Verification items for the finished model (mm, model axes). A direction names the side the tool comes from. Give positions to 0.01 mm unless a question says otherwise; leave off trailing zeros. Loops run counter-clockwise (first coordinate to the right, second up) from the corner with the lowest first, then second, coordinate; pieces in that order, holes last. Notation, with made-up numbers: (-26, -8.5) - (-8, -8.5) arc R14 cw to (-8, 4.5) - close; hole circle Ø4 at (58.25, 78.5). An arc over 180 degrees is marked (long way). Answer in a Markdown table with one row per item.
```python
from build123d import *

# Parameters (mm, degrees)
SKETCH1_W                          = 38.1
SKETCH1_H                          = 63.5
MAIN_BODY_DEPTH                    = 3.175
SKETCH2_W                          = 3.2258
SKETCH2_H                          = 6.35
TABS_DEPTH                         = 3.175
SKETCH5_R                          = 0.508
MOTOR_CUT_DEPTH                    = 4.175
SKETCH6_R                          = 3.2385
CUT_FOR_AXLE_DEPTH                 = 4.175
ROUND_OFF_BACK_CORNER_DEPTH        = 4.175
SKETCH8_W                          = 3.2258
SKETCH8_H                          = 6.35
CUT_FOR_TABS_DEPTH                 = 4.175
SKETCH9_R                          = 1.5875
CUT_FOR_BRACKET_SCREW_DEPTH        = 4.175
SKETCH10_R                         = 3.048
CUT_FOR_BASIC_2ND_MOUNT_AXLE_DEPTH = 4.175
SKETCH11_W                         = 9.398
SKETCH11_H                         = 5.08
CUT_EXTRUDE1_DEPTH                 = 4.175


with BuildPart() as part:
    # Sketch1 → main body (new body)
    with BuildSketch(Plane(origin=(0, 0, 0), x_dir=(0, 0, -1), z_dir=(1, 0, 0))):
        Rectangle(SKETCH1_W, SKETCH1_H)
    extrude(amount=MAIN_BODY_DEPTH)

    # Sketch2 → tabs (add)
    with BuildSketch(Plane(origin=(3.175, 0, 0), x_dir=(0, 0, -1), z_dir=(1, 0, 0))):
        with Locations((-20.6629, 22.225)):
            Rectangle(SKETCH2_W, SKETCH2_H)
        with Locations((-20.6629, -3.175)):
            Rectangle(SKETCH2_W, SKETCH2_H)
    extrude(amount=-TABS_DEPTH)

    # Sketch5 → motor cut (cut, through all)
    with BuildSketch(Plane(origin=(3.175, 0, 0), x_dir=(0, 0, -1), z_dir=(1, 0, 0))):
        with Locations((1.905, -28.956)):
            Circle(SKETCH5_R)
        with Locations((1.905, -1.016)):
            Circle(SKETCH5_R)
        Polygon((8.255, -3.556), (-4.445, -3.556), (-4.445, -26.416), (-1.27, -26.416), (-1.27, -27.813), (5.08, -27.813), (5.08, -26.416), (8.255, -26.416), align=None)
    extrude(amount=-MOTOR_CUT_DEPTH, mode=Mode.SUBTRACT)

    # Sketch6 → cut for axle (cut, through all)
    with BuildSketch(Plane(origin=(3.175, 0, 0), x_dir=(0, 0, -1), z_dir=(1, 0, 0))):
        with Locations((-1.27, 23.495)):
            Circle(SKETCH6_R)
    extrude(amount=-CUT_FOR_AXLE_DEPTH, mode=Mode.SUBTRACT)

    # Sketch7 → round off back corner (cut, through all)
    with BuildSketch(Plane(origin=(3.175, 0, 0), x_dir=(0, 0, -1), z_dir=(1, 0, 0))):
        with BuildLine():
            Line((19.05, -31.75), (19.05, -6.35))
            ThreePointArc((19.05, -6.35), (15.925359096, -20.215661593), (7.62, -31.75))
            Line((7.62, -31.75), (19.05, -31.75))
        make_face()
    extrude(amount=-ROUND_OFF_BACK_CORNER_DEPTH, mode=Mode.SUBTRACT)

    # Sketch8 → cut for tabs (cut, through all)
    with BuildSketch(Plane(origin=(3.175, 0, 0), x_dir=(0, 0, -1), z_dir=(1, 0, 0))):
        with Locations((14.2113, 22.225)):
            Rectangle(SKETCH8_W, SKETCH8_H)
        with Locations((14.2113, 6.985)):
            Rectangle(SKETCH8_W, SKETCH8_H)
    extrude(amount=-CUT_FOR_TABS_DEPTH, mode=Mode.SUBTRACT)

    # Sketch9 → cut for bracket screw (cut, through all)
    with BuildSketch(Plane(origin=(3.175, 0, 0), x_dir=(0, 0, -1), z_dir=(1, 0, 0))):
        with Locations((-12.7, 15.24)):
            Circle(SKETCH9_R)
    extrude(amount=-CUT_FOR_BRACKET_SCREW_DEPTH, mode=Mode.SUBTRACT)

    # Sketch10 → cut for basic 2nd mount axle (cut, through all)
    with BuildSketch(Plane(origin=(3.175, 0, 0), x_dir=(0, 0, -1), z_dir=(1, 0, 0))):
        with Locations((-11.43, -1.27)):
            Circle(SKETCH10_R)
    extrude(amount=-CUT_FOR_BASIC_2ND_MOUNT_AXLE_DEPTH, mode=Mode.SUBTRACT)

    # Sketch11 → Cut-Extrude1 (cut, through all)
    with BuildSketch(Plane(origin=(3.175, 0, 0), x_dir=(0, 0, -1), z_dir=(1, 0, 0))):
        with Locations((-8.001, 7.630964138)):
            Rectangle(SKETCH11_W, SKETCH11_H)
    extrude(amount=-CUT_EXTRUDE1_DEPTH, mode=Mode.SUBTRACT)


solid = part.part
```
Q1. Sectioned sample at C-C (z = 2). Record the cut outline in (x, y) (3 decimals).
Completed:
| item | result |
|---|---|
| outline | (0, -31.75) - (3.175, -31.75) - (3.175, -26.416) - (0, -26.416) - close; (0, -3.556) - (3.175, -3.556) - (3.175, 20.34) - (0, 20.34) - close; (0, 26.65) - (3.175, 26.65) - (3.175, 31.75) - (0, 31.75) - close |
Q2. Sectioned sample at D-D (y = 24.5). Record the cut outline in (x, z) (3 decimals), and give its area (3 significant figures).
Completed:
| item | result |
|---|---|
| outline | (0, -19.05) - (3.175, -19.05) - (3.175, -15.824) - (0, -15.824) - close; (0, -12.598) - (3.175, -12.598) - (3.175, -1.809) - (0, -1.809) - close; (0, 4.349) - (3.175, 4.349) - (3.175, 22.276) - (0, 22.276) - close |
| area | 101 mm^2 |
Q3. Go/stop test with flat-tipped pins: P1, Ø1, axis at x = 2.5, y = 6, coming from the +Z side; P2, Ø0.6, axis at y = -1.016, z = -1.905, coming from the +X side; P3, Ø1.6, axis at x = 1, z = 21, coming from the +Y side; P4, Ø1.5, axis at x = 1.5, y = -27, coming from the -Z side. Record where each tip stops, or that it passes through.
Completed:
| item | result |
|---|---|
| P1 | z = 19.05 |
| P2 | through |
| P3 | y = 25.4 |
| P4 | z = -12.46 |
Q4. Draft check along Y on faces 1 (the face through (2, -3, 22.276)), 2 (the face through (1.61, 26.706, 1.692)), 3 (the face through (2, -6.35, 21)). Enter one of: +Y half, -Y half, draft (parallel to the pull), parting line (faces both ways), or undercut.
Completed:
| item | result |
|---|---|
| face 1 | draft |
| face 2 | undercut |
| face 3 | -Y half |
Q5. Sectioned sample at B-B (z = -7). Record the cut outline in (x, y) (3 decimals).
Completed:
| item | result |
|---|---|
| outline | (0, -31.75) - (3.175, -31.75) - (3.175, -26.416) - (0, -26.416) - close; (0, -3.556) - (3.175, -3.556) - (3.175, 31.75) - (0, 31.75) - close |
Q6. Tool access check on faces 4 (the face through (2, -19, 19.05)), 5 (the face through (2, 22, 22.276)), 6 (the face through (2, -15, -8.255)), 7 (the face through (2, 19.05, 21)). Record the directions out of +Z, -Z, +X, -X, +Y, -Y that give a thin tool (end or side, any length) a straight path to the whole face; none if there is none.
Completed:
| item | result |
|---|---|
| face 4 | +Z, +X, -X, -Y |
| face 5 | +Z, +X, -X, +Y, -Y |
| face 6 | +X, -X |
| face 7 | +Z, +X, -X |
Q7. Thickness scan on line 1 (Y direction, x = 0.4, z = 12); line 2 (Y direction, x = 1.65, z = 20); line 3 (Y direction, x = 0.4, z = 14). Record the ranges inside material, lowest first.
Completed:
| item | result |
|---|---|
| line 1 | -31.75 to -4.26, 1.72 to 5.09, 10.17 to 13.82, 16.66 to 31.75 |
| line 2 | -6.35 to 0, 19.05 to 25.4 |
| line 3 | -31.75 to -2.91, 0.37 to 14.33, 16.15 to 31.75 |
